Geometry: final body of the model. Coordinates: model frame, mm. Give positions to 0.01 mm unless a question says otherwise; leave off trailing zeros. Write each loop counter-clockwise with the first axis right and the second up, starting at its lowest first coordinate (ties: lowest second). Pieces come first, ordered by that corner, then holes.
Q1. Line query: L1, parallel to Y at x = 12.7, z = -6.5; L2, parallel to X at y = 2.5, z = -6.25; L3, parallel to Z at x = 6.25, y = 3.5. Output: solid intervals per line, ascending.
Q2. Cut plane B-B on z = -6.35. Return the cut outline in (x, y), plus the area to 3 significant figures.
Q3. Draft query along X for faces 1 (the face through (9, 12.7, -6)), 2 (the face through (19.05, 6, -6)), 3 (the face through (6.976, 6.261, -4.363)). Return one class per face: pulls with the +X half, pulls with the -X half, needs draft (parallel to the pull), parting line crosses it, or undercut.
Q4. Cut plane A-A on y = 6.35. Return the cut outline in (x, z).
Q5. Cut plane C-C on x = 12.7. Return the cut outline in (y, z).
Q6. Pin query (flat end, axial travel): pin 1 (3.5 mm diameter, centred on x = 12.7, y = 6.35, fed in from +Z). Return the tip coordinate at first contact, or that it passes through.
Q7. Cut plane D-D on y = 1. Return the cut outline in (x, z), plus the area to 3 significant figures.
```python
from build123d import *

# Parameters (mm, degrees)
SKETCH1_W           = 19.05
SKETCH1_H           = 12.7
SKETCH1_R           = 2.0828
BOSS_EXTRUDE1_DEPTH = 12.7
SKETCH2_R           = 2.0828
CUT_EXTRUDE1_DEPTH  = 12.7


with BuildPart() as part:
    # Sketch1 → Boss-Extrude1 (new body)
    with BuildSketch(Plane(origin=(0, 0, 0), x_dir=(1, 0, 0), z_dir=(0, 1, 0))):
        with Locations((9.525, 6.35)):
            Rectangle(SKETCH1_W, SKETCH1_H)
        with Locations(Location((6.35, 6.35, 0), (0, 0, 270))):
            Circle(SKETCH1_R, mode=Mode.SUBTRACT)
    extrude(amount=BOSS_EXTRUDE1_DEPTH)

    # Sketch2 → Cut-Extrude1 (cut)
    with BuildSketch(Plane.XY):
        with Locations((12.7, 6.35)):
            Circle(SKETCH2_R)
    extrude(amount=-CUT_EXTRUDE1_DEPTH, mode=Mode.SUBTRACT)


solid = part.part
```
Data:
1. L1: y = 0 to 4.27, 8.43 to 12.7
1. L2: x = 0 to 4.27, 8.43 to 19.05
1. L3: z = -12.7 to -8.43, -4.27 to 0
2. outline: (0, 0) - (4.27, 0) - (4.27, 12.7) - (0, 12.7) - close; (8.43, 0) - (19.05, 0) - (19.05, 12.7) - (8.43, 12.7) - close; hole circle Ø4.17 at (12.7, 6.35)
2. area: 175 mm2
3. face 1: needs draft
3. face 2: pulls with the +X half
3. face 3: undercut
4. outline: (0, -12.7) - (10.62, -12.7) - (10.62, 0) - (0, 0) - close; (14.78, -12.7) - (19.05, -12.7) - (19.05, 0) - (14.78, 0) - close; hole circle Ø4.17 at (6.35, -6.35)
5. outline: (0, -12.7) - (4.27, -12.7) - (4.27, 0) - (0, 0) - close; (8.43, -12.7) - (12.7, -12.7) - (12.7, 0) - (8.43, 0) - close
6. pin 1: passes through
7. outline: (0, -12.7) - (19.05, -12.7) - (19.05, 0) - (0, 0) - close; hole circle Ø4.17 at (6.35, -6.35)
7. area: 228 mm2
